Could you check a few things on this model? Use its own coordinates, in mm. Face numbers are marked on the shaded views. A direction names the side the tool comes from. Coordinates: 2 decimals unless noted, no trailing zeros. Order: outer loops, then holes, each group sorted by start corner. A loop starts at its lowest first (then second) coordinate and runs counter-clockwise, first axis right, second up. Notation, with made-up numbers: (5.25, 30.25) - (42.25, 30.25) arc R18 cw to (42.25, 35.25) - close; hole circle Ø10 at (45.25, 81). An arc over 180 degrees is marked (long way). Answer as CSV lines item,"result". Start each with the question number.
1. I want a section at C-C, the plane x = 24.5. List the corners of the cut face in (y, z) for me, and give its area (3 significant figures).
2. I want a section at B-B, the plane y = 0. List the corners of the cut face in (x, z) for me.
3. For the marked faces 1 and 2, which set-ups out of +Z, -Z, +X, -X, +Y, -Y let a thin tool reach every point of the face, with its end or its side?
4. I need wall thicknesses on probe 1 along Y at (x, z) = (33, 0); probe 2 along X at (y, z) = (1.5, -0.25); probe 3 along X at (y, z) = (-2, -2.5). Which ranges of each line are inside material? Lowest first, please.
5. I want a section at A-A, the plane z = 0. List the corners of the cut face in (x, y) for me.
6. For pin 1 (1.5 mm diameter, centred on x = 35, z = -1, fed in from +Y); pin 2 (2 mm diameter, centred on y = -0.5, z = 0, fed in from -X); pin 3 (2 mm diameter, centred on x = 1, y = 1.5, fed in from +Z); pin 4 (2 mm diameter, centred on x = 1, y = 1, fed in from -Z), each with a flat end and sliding along its axis, tell me the tip position at first contact or that it passes through.
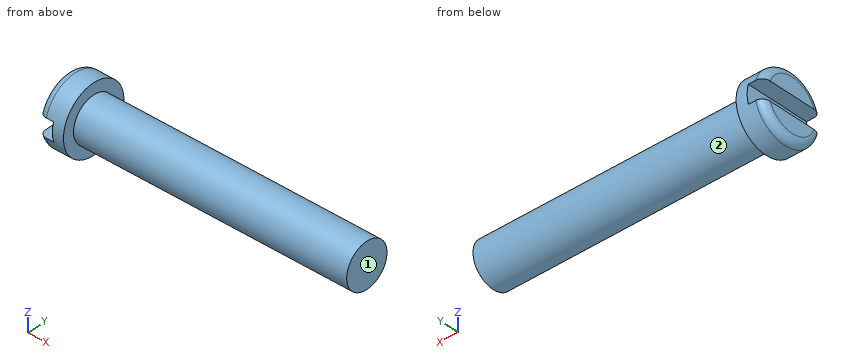
Autodesk Inventor part; units mm, degrees
ref_plane "YZ Plane" through (0, 0, 0) normal (1, 0, 0) x (0, 1, 0)
ref_plane "XZ Plane" through (0, 0, 0) normal (0, 1, 0) x (-1, 0, 0)
ref_plane "XY Plane" through (0, 0, 0) normal (0, 0, 1) x (1, 0, 0)
sketch "Skizze1" plane through (0, 0, 0) normal (0, 1, 0) x (-1, 0, 0)
  line L0 (0, 0) -> (0, 4.5)
  line L1 (0, 4.5) -> (-3.5, 4.5)
  line L2 (-3.5, 4.5) -> (-3.5, 3)
  line L3 (-3.5, 3) -> (-40.5, 3)
  line L4 (-40.5, 3) -> (-40.5, 0)
  line L5 (-40.5, 0) -> (0, 0)
  dimension "d0" = 3.5
  dimension "d1" = 6
  dimension "d2" = 9
  dimension "d3" = 37
revolve "Umdrehung1" add sketch "Skizze1" angle 360 about axis through (40.5, 0, 0) along (-1, 0, 0)
thread "Gewinde1"
sketch "Skizze2" plane through (0, 0, 0) normal (-1, 0, 0) x (0, 0, 1)
  line L0 (1.25, 4.3229) -> (1.25, -4.3229)
  line L1 (-1.25, -4.3229) -> (-1.25, 4.3229)
  circle A0 centre (0, 0) radius 4.5
  line L2 (0, 4.5) -> (0, -4.5) construction
  point P0 (0, 0)
  dimension "d7" = 2.5
extrude "Extrusion1" cut sketch "Skizze2" against normal blind 2 contours L0 A0 L1
fillet "Rundung1" radius 1 3 edges at (0, 2.7042, 3.5969) (0, -2.7042, 3.5969) (0, 0, -4.5)
properties part number "screw" material "Steel, Cast"
Solved:
1,outline,"circle Ø6 at (0, 0)"
1,area,"28.3 mm2"
2,outline,"(0, -3.5) arc R1 ccw to (1, -4.5) - (3.5, -4.5) - (3.5, -3) - (40.5, -3) - (40.5, 3) - (3.5, 3) - (3.5, 4.5) - (1, 4.5) arc R1 ccw to (0, 3.5) - (0, 1.25) - (2, 1.25) - (2, -1.25) - (0, -1.25) - close"
3,face 1,"+Z, -Z, +X, +Y, -Y"
3,face 2,"+X"
4,probe 1,"y = -3 to 3"
4,probe 2,"x = 2 to 40.5"
4,probe 3,"x = 0 to 3.5"
5,outline,"(2, -4.5) - (3.5, -4.5) - (3.5, -3) - (40.5, -3) - (40.5, 3) - (3.5, 3) - (3.5, 4.5) - (2, 4.5) - close"
6,pin 1,"stops at y = 2.99"
6,pin 2,"stops at x = 2"
6,pin 3,"stops at z = 4.47"
6,pin 4,"stops at z = -4.5"
